Here's how the part is built. I have some questions about the finished solid (model axes, mm). A direction names the side the tool comes from. Coordinates: 2 decimals unless noted, no trailing zeros. Loops run counter-clockwise (first coordinate to the right, second up) from the corner with the lowest first, then second, coordinate; pieces in that order, holes last. Notation, with made-up numbers: (-16, 78.25) -> (2, 78.25) arc R33 cw to (2, 114.25) -> close; hole circle Ø11 at (38, 27.5). An arc over 180 degrees is marked (long way). Use CSV: the item, a comma, the result in double quotes. Start each with the question number.
Autodesk Inventor part; units mm, degrees
ref_plane "YZ Plane" through (0, 0, 0) normal (1, 0, 0) x (0, 1, 0)
ref_plane "XZ Plane" through (0, 0, 0) normal (0, 1, 0) x (-1, 0, 0)
ref_plane "XY Plane" through (0, 0, 0) normal (0, 0, 1) x (1, 0, 0)
sketch "Sketch1" plane through (0, 0, 0) normal (0, 0, 1) x (1, 0, 0)
  circle A0 centre (13.2036, 20.3187) radius 2.0955
  circle A1 centre (-12.1964, 20.3187) radius 2.0955
  line L0 (2.9057, 25.0812) -> (-1.8984, 25.0812)
  circle A2 centre (-25.2051, 29.4175) radius 2.0955
  arc A3 (-22.7052, 33.4711) -> (-28.3391, 25.8315) centre (-25.2051, 29.4175) ccw
  arc A4 (29.3464, 25.8315) -> (23.7125, 33.4711) centre (26.2124, 29.4175) ccw
  circle A5 centre (26.2124, 29.4175) radius 2.0955
  line L1 (-22.7052, 33.4711) -> (-15.2312, 28.8619)
  line L2 (23.7125, 33.4711) -> (16.2385, 28.8619)
  arc A6 (-15.2312, 28.8619) -> (-1.8984, 25.0812) centre (-1.8984, 50.4812) ccw
  arc A7 (2.9057, 25.0812) -> (16.2385, 28.8619) centre (2.9057, 50.4812) ccw
  arc A8 (-16.4554, 15.4455) -> (-12.1964, 13.8467) centre (-12.1964, 20.3187) ccw
  arc A9 (13.2036, 13.8467) -> (17.4626, 15.4455) centre (13.2036, 20.3187) ccw
  line L3 (-12.1964, 13.8467) -> (13.2036, 13.8467)
  line L4 (-28.3391, 25.8315) -> (-16.4554, 15.4455)
  line L5 (17.4626, 15.4455) -> (29.3464, 25.8315)
  circle A10 centre (-12.1964, 20.3187) radius 3.6662
  circle A11 centre (13.2036, 20.3187) radius 3.6662
  point P0 (0, 0)
  point P1 (-12.1964, 25.0812)
  point P2 (17.4758, 18.214)
  point P3 (-16.4686, 18.214)
  point P4 (0.5036, 25.0812)
  dimension "d8" = 4.191
  dimension "d9" = 4.191
  dimension "d13" = 4.191
  dimension "d14" = 9.525
  dimension "d15" = 9.525
  dimension "d16" = 4.191
  dimension "d17" = 25.4
  dimension "d19" = 7.3323
  dimension "d21" = 15.875
  dimension "d23" = 15.875
extrude "Extrusion1" add sketch "Sketch1" along normal blind 1.5875 contours A7 L2 A4 L5 A9 L3 A8 L4 A3 L1 A6 L0 | A10 | A11
properties part number "Hook Gusset Brace" material "Acetal Resin, White"
1) Please list where these lines run through material, in increasing order: L1, parallel to X at y = 28.75, z = 1.45; L2, parallel to X at y = 18.5, z = 1.5; L3, parallel to X at y = 27.75, z = 0.1. Write a range as [from, to].
2) I want a section at B-B, the plane y = 19.75. Please give me the cut outline in (x, z).
3) I want a section at D-D, the plane x = 20.5. Please give me the cut outline in (y, z), plus the area to 3 significant figures.
4) I want a section at C-C, the plane z = 0.6. Please give me the cut outline in (x, y), plus the area to 3 significant figures.
5) Which directions (+Z, -Z, +X, -X, +Y, -Y) give clear straight access to the entire face, cutting with the end or side of a thin tool? Please do faces 1 (the face through (29.99, 32.32, 0.78)), 2 (the face through (9.93, 26.07, 0.78)).
6) Thinking about a two-plate mould opening in X: for faces 3 (the face through (-22.48, 20.71, 0.78)), 4 (the face through (20.03, 31.2, 0.78)), 5 (the face through (23.321, 20.566, 0.783)), 6 (the face through (-11.23, 22.18, 0.78)), which applies, pulls with the +X half, pulls with the -X half, needs draft (parallel to the pull), parting line crosses it, or undercut?
7) I want a section at A-A, the plane y = 28.25. Please give me the cut outline in (x, z), plus the area to 3 significant figures.
Return value:
1,L1,"x = [-29.92, -27.19], [-23.22, -15.05], [16.06, 24.23], [28.2, 30.93]"
1,L2,"x = [-19.95, -13.24], [-11.16, 12.16], [14.24, 20.96]"
1,L3,"x = [-29.67, -26.47], [-23.94, -13.23], [14.24, 24.94], [27.48, 30.67]"
2,outline,"(-21.38, 0) -> (-14.21, 0) -> (-14.21, 1.59) -> (-21.38, 1.59) -> close; (-10.18, 0) -> (11.19, 0) -> (11.19, 1.59) -> (-10.18, 1.59) -> close; (15.22, 0) -> (22.39, 0) -> (22.39, 1.59) -> (15.22, 1.59) -> close"
3,outline,"(18.1, 0) -> (31.49, 0) -> (31.49, 1.59) -> (18.1, 1.59) -> close"
3,area,"21.3 mm²"
4,outline,"(-28.34, 25.83) -> (-16.46, 15.45) arc R6.47 ccw to (-12.2, 13.85) -> (13.2, 13.85) arc R6.47 ccw to (17.46, 15.45) -> (29.35, 25.83) arc R4.76 ccw to (23.71, 33.47) -> (16.24, 28.86) arc R25.4 cw to (2.91, 25.08) -> (-1.9, 25.08) arc R25.4 cw to (-15.23, 28.86) -> (-22.71, 33.47) arc R4.76 ccw to start; hole circle Ø4.19 at (-25.21, 29.42); hole circle Ø4.19 at (-12.2, 20.32); hole circle Ø4.19 at (13.2, 20.32); hole circle Ø4.19 at (26.21, 29.42)"
4,area,"666 mm²"
5,face 1,"+Z, -Z"
5,face 2,"+Z, -Z, +Y"
6,face 3,"pulls with the -X half"
6,face 4,"undercut"
6,face 5,"pulls with the +X half"
6,face 6,"undercut"
7,outline,"(-29.82, 0) -> (-26.95, 0) -> (-26.95, 1.59) -> (-29.82, 1.59) -> close; (-23.46, 0) -> (-14.18, 0) -> (-14.18, 1.59) -> (-23.46, 1.59) -> close; (15.19, 0) -> (24.47, 0) -> (24.47, 1.59) -> (15.19, 1.59) -> close; (27.95, 0) -> (30.83, 0) -> (30.83, 1.59) -> (27.95, 1.59) -> close"
7,area,"38.6 mm²"
